CAD build for the part. Positions are in the model's coordinates, mm. Coordinates: 2 decimals unless noted, no trailing zeros. Loops run counter-clockwise (first coordinate to the right, second up) from the corner with the lowest first, then second, coordinate; pieces in that order, holes last. Notation, with made-up numbers: (-10.75, -36) -> (17.25, -36) arc R22 ccw to (17.25, -10) -> close; hole circle Ø1 at (76, 83.5). An arc over 180 degrees is marked (long way). Write each question's results on one line, items separated by ' | '.
```python
from build123d import *

# Parameters (mm, degrees)
ESQUISSE1_R        = 2.75
BOSS_EXTRU_1_DEPTH = 5
CHANFREIN1_SIZE    = 2.8


with BuildPart() as part:
    # Esquisse1 → Boss.-Extru.1 (new body)
    with BuildSketch(Plane.XY):
        with BuildLine():
            Line((0, 7), (60, 7))
            ThreePointArc((60, 7), (67, 0), (60, -7))
            Line((60, -7), (0, -7))
            ThreePointArc((0, -7), (-7, 0), (0, 7))
        make_face()
        with Locations((60, 0)):
            Circle(ESQUISSE1_R, mode=Mode.SUBTRACT)
        Circle(ESQUISSE1_R, mode=Mode.SUBTRACT)
    extrude(amount=BOSS_EXTRU_1_DEPTH)

    # Chanfrein1
    chanfrein1_edges = [part.edges().sort_by_distance(p)[0] for p in [
        (57.25, 0, 5),
        (-2.75, 0, 5),
    ]]
    chamfer(chanfrein1_edges, length=CHANFREIN1_SIZE)


solid = part.part
```
Q1. Cut at A-A on y = 0. Write the cut outline in (x, z), and give its area (3 significant figures).
Results are:
outline: (-7, 0) -> (-2.75, 0) -> (-2.75, 2.2) -> (-5.55, 5) -> (-7, 5) -> close; (2.75, 0) -> (57.25, 0) -> (57.25, 2.2) -> (54.45, 5) -> (5.55, 5) -> (2.75, 2.2) -> close; (62.75, 0) -> (67, 0) -> (67, 5) -> (65.55, 5) -> (62.75, 2.2) -> close | area: 299 mm^2
Q2. Cut at B-B on z = 4.25. Write the cut outline in (x, y), and give its area (3 significant figures).
Results are:
outline: (0, -7) -> (60, -7) arc R7 ccw to (60, 7) -> (0, 7) arc R7 ccw to start; hole circle Ø9.6 at (0, 0); hole circle Ø9.6 at (60, 0) | area: 849 mm^2
Q3. Wall check: L1, parallel to X at y = 1.5, z = 4.55; L2, parallel to Y at x = 0, z = 0.85; L3, parallel to X at y = 4.5, z = 4.55. Give the ranges that are in metal, low to high. Write a range as from..to.
Results are:
L1: -6.84..-4.87, 4.87..55.13, 64.87..66.84 | L2: -7..-2.75, 2.75..7 | L3: -5.36..-2.4, 2.4..57.6, 62.4..65.36
Q4. Pull direction Y, two halves, no side cores. Call faces 1 (the cylindrical face through (67, 0, 2)), 2 (the flat face through (30, 7, 2)), 3 (the flat face through (31, 0, 5)), 4 (the cylindrical face through (-0.596, -2.685, 1.085)): +Y half, -Y half, draft (parallel to the pull), parting line (faces both ways), or undercut.
Results are:
face 1: parting line | face 2: +Y half | face 3: draft | face 4: undercut
Q5. Drop a flat-ended pin along its axis: pin 1 (5 mm diameter, centred on x = 35.5, y = -5, fed in from -Z). Give the stop position or say it passes through.
Results are:
pin 1: z = 0
